Geometry: final body of the model. Coordinates: model frame, mm. A direction names the side the tool comes from. Give positions to 0.01 mm unless a question says otherwise; leave off trailing zeros. Write each loop counter-clockwise with the first axis right and the second up, starting at its lowest first coordinate (ties: lowest second). Pieces come first, ordered by that corner, then holes. Notation, with made-up numbers: M -14.75,21 L 22.25,21 A30 cw 22.25,57 Z; hole C 25.25,38.25 d7. An arc over 180 degrees is marked long. Use one line per item in the form item = value. Start each with the question number.
Item 1: Pull-direction query (Y, two-part tool) for faces 1 (the flat face through (1, -13, 37.522)), 2 (the cylindrical face through (1.019, -6.009, 39.423)), 3 (the flat face through (72.771, -7, -3)), 4 (the cylindrical face through (1.02, -20.07, 39.52)); classes: released by +Y, released by -Y, zero draft, split by the parting line, or undercut.
Item 2: Material intervals for line 1 along Z through (x, y) = (53, -14.25); line 2 along Y through (x, z) = (25, -15.5); line 3 along Z through (x, y) = (0, -5.1), sorted ascending. Write a range as from..to.
Item 3: Contact query for flat-ended pins moving along their axis: P1, Ø10, axis at x = -48.5, z = 24.5, coming from the -Y side; P2, Ø4, axis at x = 1, y = -21, coming from the +Z side; P3, Ø1.9, axis at x = -2.5, y = -19.5, coming from the -Z side. Output: stop coordinate, or through.
Item 4: Section query A-A on x = -31.5. Return loops of the section in (y, z).
Item 5: Access query for faces 5 (the cylindrical face through (1.019, -6.108, -39.521)), 6 (the flat face through (1, -18.168, 35)). Directions: +Z, -Z, +X, -X, +Y, -Y. A direction counts if a zero-diameter tool reaches every point of the face in a straight line with its end or side. Return the directions, or none.
Item 6: Section query B-B on z = 22. Return loops of the section in (x, y).
from build123d import *

# Parameters (mm, degrees)
F1_DEPTH      = 72.771
F1_DEPTH_BACK = 72.771
F2_R          = 0.9525
F3_DEPTH      = 2.794


# Not quite as in the source:
# - a length typed as a fraction of an inch, garbled in the dataset ("3 / 203.2 mm" for 3/8 in), is restored


with BuildPart() as f1:
    # F0 (on Right) → F1 (new body, two sides)
    with BuildSketch(Plane.YZ) as f1_sk:
        with BuildLine():
            Line((-8.008403407, 37.52215), (-8.008403407, 0))
            Line((-8.008403407, 0), (-8.008403407, -37.52215))
            Line((-8.008403407, -37.52215), (-18.168403407, -37.52215))
            Line((-18.168403407, -37.52215), (-18.168403407, -32.69615))
            Line((-18.168403407, -32.69615), (-21.978403407, -32.69615))
            Line((-21.978403407, -32.69615), (-21.978403407, -34.98215))
            ThreePointArc((-21.978403407, -34.98215), (-20.1185314675, -39.4722780605), (-15.628403407, -41.33215))
            Line((-15.628403407, -41.33215), (-10.548403407, -41.33215))
            ThreePointArc((-10.548403407, -41.33215), (-6.0582753465, -39.4722780605), (-4.198403407, -34.98215))
            Line((-4.198403407, -34.98215), (-4.198403407, 0))
            Line((-4.198403407, 0), (-4.198403407, 34.98215))
            ThreePointArc((-4.198403407, 34.98215), (-6.0582753465, 39.4722780605), (-10.548403407, 41.33215))
            Line((-10.548403407, 41.33215), (-15.628403407, 41.33215))
            ThreePointArc((-15.628403407, 41.33215), (-20.1185314675, 39.4722780605), (-21.978403407, 34.98215))
            Line((-21.978403407, 34.98215), (-21.978403407, 32.69615))
            Line((-21.978403407, 32.69615), (-18.168403407, 32.69615))
            Line((-18.168403407, 32.69615), (-18.168403407, 37.52215))
            Line((-18.168403407, 37.52215), (-8.008403407, 37.52215))
        make_face()
    extrude(amount=F1_DEPTH)
    extrude(f1_sk.sketch, amount=-F1_DEPTH_BACK)

    # F2 (on face) → F3 (cut)
    with BuildSketch(Plane(origin=(0, -4.198403407, 0), x_dir=(-1, 0, 0), z_dir=(0, 1, 0))):
        Circle(F2_R)
    extrude(amount=-F3_DEPTH, mode=Mode.SUBTRACT)


solid = f1.part
Answer sheet:
q1.face_1 = undercut
q1.face_2 = released by +Y
q1.face_3 = zero draft
q1.face_4 = released by -Y
q2.line_1 = -41.33..-37.52, 37.52..41.33
q2.line_2 = -8.01..-4.2
q2.line_3 = -38.24..-0.95, 0.95..38.24
q3.P1 = -8.01
q3.P2 = 40.36
q3.P3 = -40.62
q4.outline = M -21.98,-34.98 A6.35 ccw -15.63,-41.33 L -10.55,-41.33 A6.35 ccw -4.2,-34.98 L -4.2,34.98 A6.35 ccw -10.55,41.33 L -15.63,41.33 A6.35 ccw -21.98,34.98 L -21.98,32.7 L -18.17,32.7 L -18.17,37.52 L -8.01,37.52 L -8.01,-37.52 L -18.17,-37.52 L -18.17,-32.7 L -21.98,-32.7 Z
q5.face_5 = -Z, +X, -X, +Y
q5.face_6 = +X, -X
q6.outline = M -72.77,-8.01 L 72.77,-8.01 L 72.77,-4.2 L -72.77,-4.2 Z
